Here's how the part is built. I have some questions about the finished solid (model axes, mm). Round coordinates to 2 decimals unless told otherwise and drop trailing zeros. Write each loop counter-clockwise with the first axis right and the second up, starting at its lowest first coordinate (ties: lowest second). Pieces come first, ordered by that corner, then holes. Notation, with made-up numbers: (-27.75, 88.25) - (-5.75, 88.25) arc R9 ccw to (-5.75, 105.25) - close; hole circle Ø1 at (63, 48.5). An arc over 180 degrees is marked (long way). One line per question, with ' | ' between items. Start each with the question number.
(1) Thinking about a two-plate mould opening in Z: for faces 1 (the cylindrical face through (-55.59, -12.52, 50.98)), 2 (the cylindrical face through (-2.592, -12.878, 42.635)), 3 (the flat face through (16, -25.4, -32)), which applies, pulls with the +Z half, pulls with the -Z half, needs draft (parallel to the pull), parting line crosses it, or undercut?
(2) Imagine slicing it at C-C (z = 50). Write out the boundary of the cut face in (x, y).
(3) Imagine slicing it at D-D (y = -3.25). Write out the boundary of the cut face in (x, z).
(4) Imagine slicing it at B-B (x = 0). Write out the boundary of the cut face in (y, z), plus the area to 3 significant figures.
(5) Imagine slicing it at A-A (z = 0). Write out the boundary of the cut face in (x, y), plus the area to 3 significant figures.
(6) Will these pins go through, and if not, where does the flat tip stop? pin 1 (4 mm diameter, centred on x = 12.5, z = 25.5, fed in from -Y); pin 2 (1 mm diameter, centred on y = -10, z = -49, fed in from -X); pin 3 (6 mm diameter, centred on y = -2.5, z = 23.5, fed in from -X).
(7) If I drill on L1, parallel to Z at x = 0, y = -18.75; L2, parallel to X at y = -16.5, z = 17.5; L3, parallel to X at y = -15.25, z = -62, over which ranges is the centre line in solid material (lowest first)?
from build123d import *

# Parameters (mm, degrees)
F0_R     = 75.4260527683
F1_DEPTH = 25.4
F2_R     = 25.3745556146
F3_R     = 28.4988575913
F4_DEPTH = 80.4947149009
F6_SIZE  = 5
F7_R     = 11.9569521578
F5_DEPTH = 25.401


with BuildPart() as f1:
    # F0 (on Front) → F1 (new body)
    with BuildSketch(Plane.XZ):
        Circle(F0_R)
    extrude(amount=F1_DEPTH)

    # F2 (on face) + F3 (on face) → F4 (cut)
    with BuildSketch(Plane.XZ.offset(25.4)):
        Circle(F2_R)
    with BuildSketch(Plane.XZ.offset(25.4)):
        Circle(F3_R)
    extrude(amount=-F4_DEPTH, mode=Mode.SUBTRACT)

    # F6
    f6_edges = [f1.edges().sort_by_distance(p)[0] for p in [
        (-28.498858, -25.4, 0),
        (28.498858, -12.7, 0),
        (-28.498858, 0, 0),
    ]]
    chamfer(f6_edges, length=F6_SIZE)

    # F7 (on face) → F5 (cut, through all)
    with BuildSketch(Plane.XZ.offset(25.4)):
        with Locations((0, 54.307743907)):
            Circle(F7_R)
    extrude(amount=-F5_DEPTH, mode=Mode.SUBTRACT)


solid = f1.part
Check sheet entries:
1) face 1: parting line crosses it | face 2: undercut | face 3: needs draft
2) outline: (-56.47, -25.4) - (-11.15, -25.4) - (-11.15, 0) - (-56.47, 0) - close; (11.15, -25.4) - (56.47, -25.4) - (56.47, 0) - (11.15, 0) - close
3) outline: circle Ø150.85 at (0, 0); hole circle Ø60.5 at (0, 0); hole circle Ø23.91 at (0, 54.31)
4) outline: (-25.4, -75.43) - (0, -75.43) - (0, -33.5) - (-5, -28.5) - (-20.4, -28.5) - (-25.4, -33.5) - close; (-25.4, 33.5) - (-20.4, 28.5) - (-5, 28.5) - (0, 33.5) - (0, 42.35) - (-25.4, 42.35) - close; (-25.4, 66.26) - (0, 66.26) - (0, 75.43) - (-25.4, 75.43) - close | area: 1,730 mm^2
5) outline: (-75.43, -25.4) - (-33.5, -25.4) - (-28.5, -20.4) - (-28.5, -5) - (-33.5, 0) - (-75.43, 0) - close; (28.5, -20.4) - (33.5, -25.4) - (75.43, -25.4) - (75.43, 0) - (33.5, 0) - (28.5, -5) - close | area: 2,330 mm^2
6) pin 1: y = -22.3 | pin 2: x = -57.77 | pin 3: x = -72.59
7) L1: -75.43 to -28.5, 28.5 to 42.35, 66.26 to 75.43 | L2: -73.37 to -22.49, 22.49 to 73.37 | L3: -42.95 to 42.95
